Part print with two shaded views. Sizes in mm from the minimum x, y, z corner. Round coordinates to 2 decimals unless told otherwise and drop trailing zeros. Write each loop counter-clockwise with the first axis right and the second up, starting at its lowest first coordinate (ties: lowest second). Pieces come first, ordered by that corner, then holes. Notation, with made-up numbers: (54.25, -8.75) -> (75.25, -8.75) arc R21 cw to (75.25, 19.25) -> close; hole circle Ø6 at (42.5, 87.5). An arc over 180 degrees is marked (long way). Answer in a Markdown table with one row per item. Add a question column.
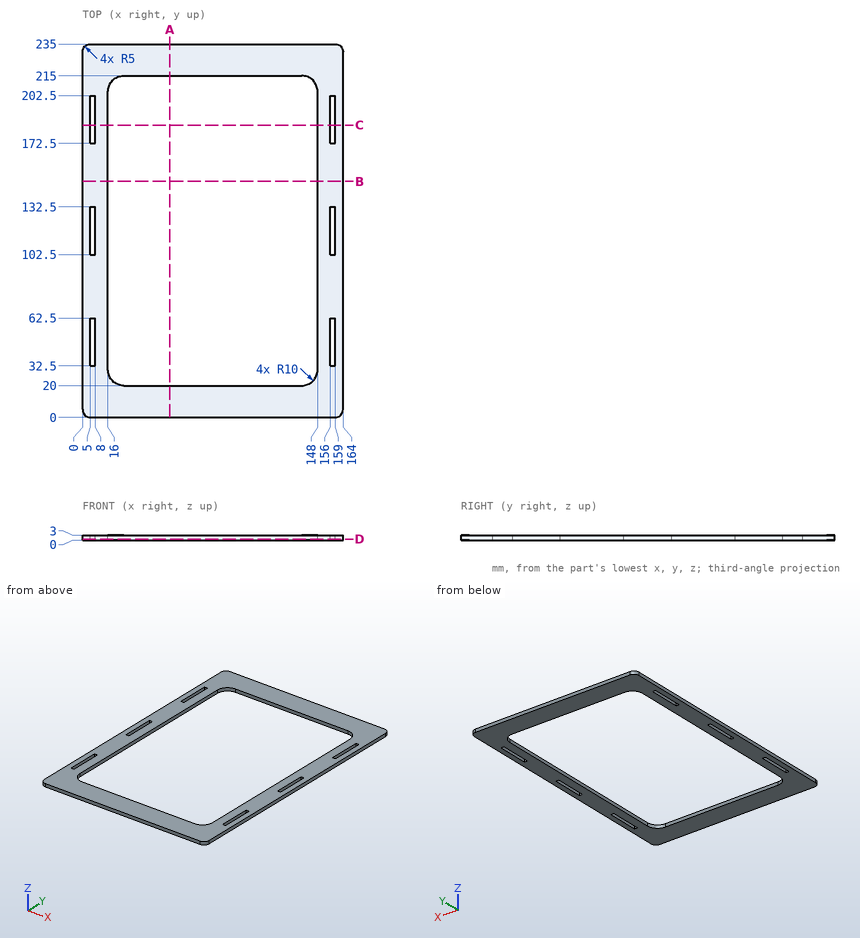
Item 1: Saw through at B-B on y = 148.5. Give the cut face in (x, z), then the cut area to 3 significant figures.
Item 2: Saw through at A-A on x = 55. Give the cut face in (y, z), then the cut area to 3 significant figures.
Item 3: Saw through at C-C on y = 184. Give the cut face in (x, z).
Item 4: Drill centre lines: probe 1 along X at (y, z) = (59, 1.45); probe 2 along Y at (x, z) = (65.5, 2.5); probe 3 along X at (y, z) = (29, 2.25). Where is each one in solid material? Low to high.
Item 5: Saw through at D-D on z = 0.7. Count the separate pieces of the cut face and the enclosed holes in it, then the cut area to 3 significant figures.
Recorded:
| question | item | result |
|---|---|---|
| 1 | outline | (0, 0) -> (16, 0) -> (16, 3) -> (0, 3) -> close; (148, 0) -> (164, 0) -> (164, 3) -> (148, 3) -> close |
| 1 | area | 96.0 mm2 |
| 2 | outline | (0, 0) -> (20, 0) -> (20, 3) -> (0, 3) -> close; (215, 0) -> (235, 0) -> (235, 3) -> (215, 3) -> close |
| 2 | area | 120 mm2 |
| 3 | outline | (0, 0) -> (5, 0) -> (5, 3) -> (0, 3) -> close; (8, 0) -> (16, 0) -> (16, 3) -> (8, 3) -> close; (148, 0) -> (156, 0) -> (156, 3) -> (148, 3) -> close; (159, 0) -> (164, 0) -> (164, 3) -> (159, 3) -> close |
| 4 | probe 1 | 0 to 5, 8 to 16, 148 to 156, 159 to 164 |
| 4 | probe 2 | 0 to 20, 215 to 235 |
| 4 | probe 3 | 0 to 16.05, 147.95 to 164 |
| 5 | separate pieces | 1 |
| 5 | enclosed holes | 7 |
| 5 | area | 12,300 mm2 |
